Part model, mm, in its own coordinate system. A direction names the side the tool comes from. Round coordinates to 2 decimals unless told otherwise and drop trailing zeros. Write each loop counter-clockwise with the first axis right and the second up, starting at its lowest first coordinate (ties: lowest second). Pieces come first, ordered by that corner, then holes.
```python
from build123d import *

# Parameters (mm, degrees)
SKETCH1_W           = 115
SKETCH1_H           = 75
SKETCH1_R           = 4.15
BOSS_EXTRUDE1_DEPTH = 5
FILLET1_R           = 20
SKETCH5_R           = 4.15
CUT_EXTRUDE4_DEPTH  = 10
CUT_EXTRUDE7_DEPTH  = 16
SKETCH12_R          = 20
CUT_EXTRUDE8_DEPTH  = 10
FILLET2_R           = 3


with BuildPart() as part:
    # Sketch1 → Boss-Extrude1 (new body)
    with BuildSketch(Plane(origin=(0, 0, 0), x_dir=(1, 0, 0), z_dir=(0, 1, 0))):
        Rectangle(SKETCH1_W, SKETCH1_H)
        with Locations(Location((-44.48, 24.48, 0), (0, 0, 270))):
            Circle(SKETCH1_R, mode=Mode.SUBTRACT)
    extrude(amount=BOSS_EXTRUDE1_DEPTH)

    # Fillet1
    fillet1_edges = [part.edges().sort_by_distance(p)[0] for p in [
        (57.5, 2.5, 37.5),
        (-57.5, 2.5, 37.5),
        (-57.5, 2.5, -37.5),
        (57.5, 2.5, -37.5),
    ]]
    fillet(fillet1_edges, radius=FILLET1_R)

    # Sketch5 → Cut-Extrude4 (cut)
    with BuildSketch(Plane.XZ):
        with Locations(Location((-39.5, 25.5, 0), (0, 0, 270))):
            Circle(SKETCH5_R)
        with Locations(Location((39.5, -25.5, 0), (0, 0, 270))):
            Circle(SKETCH5_R)
    extrude(amount=-CUT_EXTRUDE4_DEPTH, mode=Mode.SUBTRACT)

    # Sketch11 → Cut-Extrude7 (cut)
    with BuildSketch(Plane(origin=(0, 5, 0), x_dir=(1, 0, 0), z_dir=(0, 1, 0))):
        with BuildLine():
            Line((57.5, -17.5), (57.5, 17.5))
            ThreePointArc((57.5, 17.5), (51.642135624, 31.642135624), (37.5, 37.5))
            Line((37.5, 37.5), (-37.5, 37.5))
            ThreePointArc((-37.5, 37.5), (-51.642135624, 31.642135624), (-57.5, 17.5))
            Line((-57.5, 17.5), (-57.5, -17.5))
            ThreePointArc((-57.5, -17.5), (-51.642135624, -31.642135624), (-37.5, -37.5))
            Line((-37.5, -37.5), (37.5, -37.5))
            ThreePointArc((37.5, -37.5), (51.642135624, -31.642135624), (57.5, -17.5))
        make_face()
        with BuildLine():
            Line((37.5, 36.5), (-37.5, 36.5))
            ThreePointArc((-37.5, 36.5), (-50.935028843, 30.935028843), (-56.5, 17.5))
            Line((-56.5, 17.5), (-56.5, -17.5))
            ThreePointArc((-56.5, -17.5), (-50.935028843, -30.935028843), (-37.5, -36.5))
            Line((-37.5, -36.5), (37.5, -36.5))
            ThreePointArc((37.5, -36.5), (50.935028843, -30.935028843), (56.5, -17.5))
            Line((56.5, -17.5), (56.5, 17.5))
            ThreePointArc((56.5, 17.5), (50.935028843, 30.935028843), (37.5, 36.5))
        make_face(mode=Mode.SUBTRACT)
    extrude(amount=-CUT_EXTRUDE7_DEPTH, mode=Mode.SUBTRACT)

    # Sketch12 → Cut-Extrude8 (cut)
    with BuildSketch(Plane(origin=(0, 5, 0), x_dir=(1, 0, 0), z_dir=(0, 1, 0))):
        with Locations(Location((0, 0, 0), (0, 0, 270))):
            Circle(SKETCH12_R)
        with BuildLine():
            Line((0, 30.5), (0, 27.5))
            ThreePointArc((0, 27.5), (19.445436483, 19.445436483), (27.5, 0))
            Line((27.5, 0), (30.5, 0))
            ThreePointArc((30.5, 0), (21.566756826, 21.566756826), (0, 30.5))
        make_face()
        with BuildLine():
            Line((-30.5, 0), (-27.5, 0))
            ThreePointArc((-27.5, 0), (-22.707377656, 15.512092057), (-10, 25.617376915))
            Line((-10, 25.617376915), (-10, 28.814059068))
            ThreePointArc((-10, 28.814059068), (-24.852062289, 17.68120471), (-30.5, 0))
        make_face()
        with BuildLine():
            Line((0, -30.5), (0, -27.5))
            ThreePointArc((0, -27.5), (-15.512092057, -22.707377656), (-25.617376915, -10))
            Line((-25.617376915, -10), (-28.814059068, -10))
            ThreePointArc((-28.814059068, -10), (-17.68120471, -24.852062289), (0, -30.5))
        make_face()
        with BuildLine():
            Line((25.617376915, -10), (28.814059068, -10))
            ThreePointArc((28.814059068, -10), (21.566756826, -21.566756826), (10, -28.814059068))
            Line((10, -28.814059068), (10, -25.617376915))
            ThreePointArc((10, -25.617376915), (19.445436483, -19.445436483), (25.617376915, -10))
        make_face()
    extrude(amount=-CUT_EXTRUDE8_DEPTH, mode=Mode.SUBTRACT)

    # Fillet2
    # the kernel refuses this fillet: 3 mm, written as the material it takes off along each edge
    with BuildSketch(Plane(origin=(0, 0, 0), x_dir=(-0.9961231139534353, 0, 0.08797011906159574), z_dir=(-0.08797011906159574, 0, -0.9961231139534353))) as fillet2_piece_1_section:
        with BuildLine():
            CenterArc((30.5 + FILLET2_R, FILLET2_R), FILLET2_R, 180, 90)
            Line((30.5, FILLET2_R), (30.5, 0))
            Line((30.5, 0), (30.5 + FILLET2_R, 0))
        make_face()
    fillet2_piece_1 = revolve(axis=Axis((0, 0, 0), (0, 1, 0)), revolution_arc=84.953159759, mode=Mode.PRIVATE)
    fillet2_piece_1 = split(fillet2_piece_1, bisect_by=Plane(origin=(-18.564957711, 0.847104703, 10), z_dir=(0, 0, 1)), keep=Keep.TOP, mode=Mode.PRIVATE)
    add(fillet2_piece_1, mode=Mode.SUBTRACT)
    with BuildSketch(Plane(origin=(0, 0, 0), x_dir=(-0.08797011906159563, 0, -0.9961231139534353), z_dir=(0.9961231139534353, 0, -0.08797011906159563))) as fillet2_piece_2_section:
        with BuildLine():
            CenterArc((30.5 + FILLET2_R, FILLET2_R), FILLET2_R, 180, 90)
            Line((30.5, FILLET2_R), (30.5, 0))
            Line((30.5, 0), (30.5 + FILLET2_R, 0))
        make_face()
    fillet2_piece_2 = revolve(axis=Axis((0, 0, 0), (0, 1, 0)), revolution_arc=84.953159759, mode=Mode.PRIVATE)
    fillet2_piece_2 = split(fillet2_piece_2, bisect_by=Plane(origin=(-10, 0.847104703, -18.564957711), z_dir=(-1, 0, 0)), keep=Keep.TOP, mode=Mode.PRIVATE)
    add(fillet2_piece_2, mode=Mode.SUBTRACT)
    with BuildSketch(Plane(origin=(0, 0, 0), x_dir=(1, 0, 0), z_dir=(0, 0, 1))) as fillet2_piece_3:
        with BuildLine():
            CenterArc((30.5 + FILLET2_R, FILLET2_R), FILLET2_R, 180, 90)
            Line((30.5, FILLET2_R), (30.5, 0))
            Line((30.5, 0), (30.5 + FILLET2_R, 0))
        make_face()
    revolve(axis=Axis((0, 0, 0), (0, 1, 0)), revolution_arc=90, mode=Mode.SUBTRACT)
    with BuildSketch(Plane(origin=(0, 0, 0), x_dir=(0.08799861930970912, 0, 0.9961205966144786), z_dir=(-0.9961205966144786, 0, 0.08799861930970912))) as fillet2_piece_4_section:
        with BuildLine():
            CenterArc((30.5 + FILLET2_R, FILLET2_R), FILLET2_R, 180, 90)
            Line((30.5, FILLET2_R), (30.5, 0))
            Line((30.5, 0), (30.5 + FILLET2_R, 0))
        make_face()
    fillet2_piece_4 = revolve(axis=Axis((0, 0, 0), (0, 1, 0)), revolution_arc=79.903040915, mode=Mode.PRIVATE)
    fillet2_piece_4 = split(fillet2_piece_4, bisect_by=Plane(origin=(10, 0.85015092, 22.167904307), z_dir=(1, 0, 0)), keep=Keep.TOP, mode=Mode.PRIVATE)
    fillet2_piece_4 = split(fillet2_piece_4, bisect_by=Plane(origin=(22.167904307, 0.85015092, 10), z_dir=(0, 0, 1)), keep=Keep.TOP, mode=Mode.PRIVATE)
    add(fillet2_piece_4, mode=Mode.SUBTRACT)
    with BuildSketch(Plane(origin=(0, 5, 0), x_dir=(-0.9961231139534353, 0, 0.08797011906159574), z_dir=(-0.08797011906159574, 0, -0.9961231139534353))) as fillet2_piece_5_section:
        with BuildLine():
            CenterArc((30.5 + FILLET2_R, -FILLET2_R), FILLET2_R, 90, 90)
            Line((30.5 + FILLET2_R, 0), (30.5, 0))
            Line((30.5, 0), (30.5, -FILLET2_R))
        make_face()
    fillet2_piece_5 = revolve(axis=Axis((0, 5, 0), (0, 1, 0)), revolution_arc=84.953159759, mode=Mode.PRIVATE)
    fillet2_piece_5 = split(fillet2_piece_5, bisect_by=Plane(origin=(-18.564957711, 4.152895297, 10), z_dir=(0, 0, 1)), keep=Keep.TOP, mode=Mode.PRIVATE)
    add(fillet2_piece_5, mode=Mode.SUBTRACT)
    with BuildSketch(Plane(origin=(0, 5, 0), x_dir=(-0.08797011906159553, 0, -0.9961231139534353), z_dir=(0.9961231139534353, 0, -0.08797011906159553))) as fillet2_piece_6_section:
        with BuildLine():
            CenterArc((30.5 + FILLET2_R, -FILLET2_R), FILLET2_R, 90, 90)
            Line((30.5 + FILLET2_R, 0), (30.5, 0))
            Line((30.5, 0), (30.5, -FILLET2_R))
        make_face()
    fillet2_piece_6 = revolve(axis=Axis((0, 5, 0), (0, 1, 0)), revolution_arc=84.953159759, mode=Mode.PRIVATE)
    fillet2_piece_6 = split(fillet2_piece_6, bisect_by=Plane(origin=(-10, 4.152895297, -18.564957711), z_dir=(-1, 0, 0)), keep=Keep.TOP, mode=Mode.PRIVATE)
    add(fillet2_piece_6, mode=Mode.SUBTRACT)
    with BuildSketch(Plane(origin=(0, 5, 0), x_dir=(0.9961205966144787, 0, 0.08799861930970913), z_dir=(0.08799861930970913, 0, -0.9961205966144787))) as fillet2_piece_7_section:
        with BuildLine():
            CenterArc((30.5 + FILLET2_R, FILLET2_R), FILLET2_R, 180, 90)
            Line((30.5 + FILLET2_R, 0), (30.5, 0))
            Line((30.5, 0), (30.5, FILLET2_R))
        make_face()
    fillet2_piece_7 = revolve(axis=Axis((0, 5, 0), (0, -1, 0)), revolution_arc=79.903040915, mode=Mode.PRIVATE)
    fillet2_piece_7 = split(fillet2_piece_7, bisect_by=Plane(origin=(10, 4.149849079, 22.167904307), z_dir=(1, 0, 0)), keep=Keep.TOP, mode=Mode.PRIVATE)
    fillet2_piece_7 = split(fillet2_piece_7, bisect_by=Plane(origin=(22.167904307, 4.149849079, 10), z_dir=(0, 0, 1)), keep=Keep.TOP, mode=Mode.PRIVATE)
    add(fillet2_piece_7, mode=Mode.SUBTRACT)
    with BuildSketch(Plane(origin=(0, 5, 0), x_dir=(1, 0, 0), z_dir=(0, 0, 1))) as fillet2_piece_8:
        with BuildLine():
            CenterArc((30.5 + FILLET2_R, -FILLET2_R), FILLET2_R, 90, 90)
            Line((30.5 + FILLET2_R, 0), (30.5, 0))
            Line((30.5, 0), (30.5, -FILLET2_R))
        make_face()
    revolve(axis=Axis((0, 5, 0), (0, 1, 0)), revolution_arc=90, mode=Mode.SUBTRACT)


solid = part.part
```
Q1. Cut at B-B on z = 6. Write the cut outline in (x, y).
Values follow:
outline: (-56.5, 0) - (-19.08, 0) - (-19.08, 5) - (-56.5, 5) - close; (19.08, 0) - (56.5, 0) - (56.5, 5) - (19.08, 5) - close
Q2. Cut at C-C on x = 39.5. Write the cut outline in (y, z).
Values follow:
outline: (0, -36.39) - (5, -36.39) - (5, -29.65) - (0, -29.65) - close; (0, -21.35) - (5, -21.35) - (5, 36.39) - (0, 36.39) - close
Q3. Mould opens along X. For faces 4 (the flat face through (12, 0, -17)), 5 (the cylindrical face through (-19.524, 2.535, -4.336)), 6 (the cylindrical face through (50.79, 2.54, 31.08)) say: +X half, -X half, draft (parallel to the pull), parting line (faces both ways), or undercut.
Values follow:
face 4: draft
face 5: undercut
face 6: +X half
Q4. Wall check: L1, parallel to Z at x = 11, y = 4.1; L2, parallel to Z at x = 16.5, y = 1.6; L3, parallel to X at y = 1.25, z = -24.48. Give the ranges that are in metal, low to high.
Values follow:
L1: z = -36.5 to -29.36, -25.2 to -16.7, 16.7 to 25.2, 29.36 to 36.5
L2: z = -36.5 to -26.06, -22 to -11.3, 11.3 to 22, 26.06 to 36.5
L3: x = -55.17 to -48.63, -40.33 to -19.12, -12.53 to 12.53, 19.12 to 35.48, 43.52 to 55.17
Q5. Cut at A-A on y = 3.4. State how many separate pieces and enclosed holes the cut face has, plus the area to 3 significant figures.
Values follow:
separate pieces: 1
enclosed holes: 8
area: 6,040 mm2
Q6. Which spindle directions (+Z, -Z, +X, -X, +Y, -Y) get a long thin tool onto all of the face, cutting with end or side? Do faces 1 (the cylindrical face through (-51.08, 2.54, 30.79)), 2 (the cylindrical face through (-22.837, 2.535, -15.321)), 3 (the flat face through (0, 3, -29)). Say none if no direction does.
Values follow:
face 1: +Z, -X, +Y, -Y
face 2: +Y, -Y
face 3: none
Q7. Drop flat-ended pins along their axis: pin 1 (13.5 mm diameter, centred on x = -44.48, z = -24.48, fed in from -Y); pin 2 (1.5 mm diameter, centred on y = 1.5, z = -28, fed in from -X); pin 3 (1 mm diameter, centred on y = 1.5, z = -27, fed in from -X); pin 4 (1.5 mm diameter, centred on y = 2, z = 32.5, fed in from -X). Give the stop position or say it passes through.
Values follow:
pin 1: stops at y = 0
pin 2: stops at x = -53.81
pin 3: stops at x = -54.23
pin 4: stops at x = -50.07
